Could you check a few things on this model? Use its own coordinates, in mm. A direction names the side the tool comes from. Coordinates: 2 decimals unless noted, no trailing zeros. Loops run counter-clockwise (first coordinate to the right, second up) from the corner with the lowest first, then second, coordinate; pieces in that order, holes last.
from build123d import *

# Parameters (mm, degrees)
BOSS_EXTRUDE1_DEPTH = 2.3495
CUT_EXTRUDE1_REACH  = 113.399
SKETCH3_R           = 22.225
BOSS_EXTRUDE2_DEPTH = 4.699


with BuildPart() as part:
    # Sketch1 → Boss-Extrude1 (new, symmetric)
    with BuildSketch(Plane(origin=(0, 0, 0), x_dir=(1, 0, 0), z_dir=(0, 1, 0))):
        with BuildLine():
            Line((-12.7, 57.285997997), (-12.7, -45.888631599))
            Line((-12.7, -45.888631599), (-27.099810626, -97.919151671))
            ThreePointArc((-27.099810626, -97.919151671), (0, -101.6), (27.099810626, -97.919151671))
            Line((27.099810626, -97.919151671), (12.7, -45.888631599))
            Line((12.7, -45.888631599), (12.7, 57.285997997))
            Line((12.7, 57.285997997), (23.364656325, 105.391153969))
            ThreePointArc((23.364656325, 105.391153969), (0, 107.95), (-23.364656325, 105.391153969))
            Line((-23.364656325, 105.391153969), (-12.7, 57.285997997))
        make_face()
    extrude(amount=BOSS_EXTRUDE1_DEPTH, both=True)

    # Sketch2 → Cut-Extrude1 (cut, up to next)
    with BuildSketch(Plane(origin=(0, 2.3495, 0), x_dir=(1, 0, 0), z_dir=(0, 1, 0)), mode=Mode.PRIVATE) as cut_extrude1_sk1:
        Polygon((4.7625, -2.749630657), (4.7625, 2.749630657), (0, 5.499261314), (-4.7625, 2.749630657), (-4.7625, -2.749630657), (0, -5.499261314), align=None)
    cut_extrude1_tool1 = extrude(cut_extrude1_sk1.sketch, amount=-CUT_EXTRUDE1_REACH, mode=Mode.PRIVATE) & part.part
    add(cut_extrude1_tool1.solids().sort_by_distance((0, 2.3495, 0))[0], mode=Mode.SUBTRACT)

    # Sketch3 → Boss-Extrude2 (add)
    with BuildSketch(Plane.XZ.offset(2.3495)):
        Circle(SKETCH3_R)
        Polygon((4.7625, -2.749630657), (0, -5.499261314), (-4.7625, -2.749630657), (-4.7625, 2.749630657), (0, 5.499261314), (4.7625, 2.749630657), align=None, mode=Mode.SUBTRACT)
    extrude(amount=-BOSS_EXTRUDE2_DEPTH)


solid = part.part
(1) Imagine slicing it at C-C, the plane x = 2. Write out the boundary of the cut face in (y, z).
Answers:
outline: (-2.35, -107.93) - (2.35, -107.93) - (2.35, -4.34) - (-2.35, -4.34) - close; (-2.35, 4.34) - (2.35, 4.34) - (2.35, 101.58) - (-2.35, 101.58) - close
(2) Imagine slicing it at D-D, the plane z = 32.5. Write out the boundary of the cut face in (x, y), and give its area (3 significant figures).
Answers:
outline: (-12.7, -2.35) - (12.7, -2.35) - (12.7, 2.35) - (-12.7, 2.35) - close
area: 119 mm2
(3) Imagine slicing it at B-B, the plane x = 17.5. Write out the boundary of the cut face in (y, z).
Answers:
outline: (-2.35, -106.52) - (2.35, -106.52) - (2.35, -78.94) - (-2.35, -78.94) - close; (-2.35, -13.7) - (2.35, -13.7) - (2.35, 13.7) - (-2.35, 13.7) - close; (-2.35, 63.23) - (2.35, 63.23) - (2.35, 100.08) - (-2.35, 100.08) - close
(4) For pin 1 (2.5 mm diameter, centred on y = 1, z = -43, fed in from +X); pin 2 (1.4 mm diameter, centred on y = -1, z = 33.5, fed in from -X); pin 3 (2.5 mm diameter, centred on y = -1, z = -1, fed in from +X) (3 decimals), each with a flat end and sliding along its axis, tell me the tip position at first contact or that it passes through.
Answers:
pin 1: stops at x = 12.7
pin 2: stops at x = -12.7
pin 3: stops at x = 22.225
(5) I need wall thicknesses on probe 1 along Z at (x, y) = (2, 0.85); probe 2 along X at (y, z) = (-0.2, -55); probe 3 along Z at (x, y) = (-7, -1.1). Which ranges of each line are inside material? Lowest first, please.
Answers:
probe 1: z = -107.93 to -4.34, 4.34 to 101.58
probe 2: x = -12.7 to 12.7
probe 3: z = -107.72 to 101.36
(6) Which directions (+Z, -Z, +X, -X, +Y, -Y) give clear straight access to the entire face, cutting with the end or side of a thin tool? Please do faces 1 (the face through (0.33, 0.03, -107.95)), 2 (the face through (20, 0.03, 72.27)), 3 (the face through (-12.7, 0, -38)), 4 (the face through (2.41, 0.03, -4.11)).
Answers:
face 1: -Z, +Y, -Y
face 2: +X, +Y, -Y
face 3: -X, +Y, -Y
face 4: +Y, -Y
(7) We'd pull the mould along Z, two halves only. Please class faces 5 (the face through (-0.4, 0, 101.6)), 6 (the face through (-2.41, 0.03, 4.11)), 7 (the face through (6, -2.35, -2)): +Z half, -Z half, draft (parallel to the pull), parting line (faces both ways), or undercut.
Answers:
face 5: +Z half
face 6: undercut
face 7: draft
